Geometry: final body of the model. Coordinates: model frame, mm. A direction names the side the tool comes from. Coordinates: 2 decimals unless noted, no trailing zeros. Order: outer loops, then holes, each group sorted by start corner. A loop starts at its lowest first (then second) coordinate and runs counter-clockwise, first axis right, second up. Notation, with made-up numbers: M 42,67.25 L 82,67.25 A5 ccw 82,76.25 Z; hole C 35.5,42 d7. An arc over 180 degrees is marked long. Write item = value, one per line.
Autodesk Inventor part; units mm, degrees
ref_plane "YZ Plane" through (0, 0, 0) normal (1, 0, 0) x (0, 1, 0)
ref_plane "XZ Plane" through (0, 0, 0) normal (0, 1, 0) x (-1, 0, 0)
ref_plane "XY Plane" through (0, 0, 0) normal (0, 0, 1) x (1, 0, 0)
sketch "Sketch1" plane through (0, 0, 0) normal (0, 0, 1) x (1, 0, 0)
  line L0 (0, 70) -> (80, 70)
  line L1 (80, 70) -> (80, -70)
  line L2 (80, -70) -> (0, -70)
  line L3 (0, -70) -> (0, 70)
  line L4 (40, 70) -> (40, -70) construction
  line L5 (50, 70) -> (80, 40)
  line L6 (80, -40) -> (50, -70)
  point P0 (0, 0)
  point P1 (0, 0)
  dimension "d1" = 140
  dimension "d15" = 30
  dimension "d27" = 80
  dimension "d28" = 45
extrude "Plate1" add sketch "Sketch1" along normal blind 6 contours L0 L5 L1 L6 L2 L3
sketch "Sketch3" plane through (6, -70, 0) normal (-1, 0, 0) x (0, -1, 0)
  line L0 (-140, 0) -> (0, 0)
  line L1 (0, 0) -> (0, 60)
  line L2 (0, 60) -> (-140, 60)
  line L3 (-140, 60) -> (-140, 0)
edge flange "Flange1" height 60 angle 90 thickness 6 bend radius 6 thickness toward (-1, 0, 0) relief tear relief width 6 relief depth 3 edges at (0, 0, 6) wall of the first edge with corners at (6, 70, 0) (6, -70, 0) (6, -70, 60) (6, 70, 60)
bend "Bend1"
corner "Corner1"
equation "\"d2\" = Thickness"
equation "\"d17\" = BendReliefWidth"
equation "\"d18\" = BendReliefDepth"
equation "\"d19\" = MinimumRemnant"
equation "\"d20\" = TransitionRadius"
equation "\"d23\" = BendRadius"
equation "\"d24\" = CornerReliefSize"
equation "\"d25\" = GapSize"
equation "\"d26\" = JacobiRadiusSize"
equation "\"BendRadius\" = Thickness"
equation "\"BendReliefWidth\" = Thickness"
equation "\"BendReliefDepth\" = 0.5 * Thickness"
equation "\"CornerReliefSize\" = 4 * Thickness"
equation "\"MinimumRemnant\" = 2 * Thickness"
equation "\"TransitionRadius\" = BendRadius"
equation "\"JacobiRadiusSize\" = BendRadius"
equation "\"GapSize\" = Thickness"
properties part number "PNS-0812 floor ring  strengthen"
1) Section C-C, the plane z = 46. Return loops of the section in (x, y).
Numbers:
outline = M 0,-70 L 6,-70 L 6,70 L 0,70 Z
2) Set-up query: faces 1 (the face through (65, 55, 3)), 2 (the face through (6, -1, 36)). Return all of +Z, -Z, +X, -X, +Y, -Y with unobstructed straight access to the full face (end or side cutting, diameter ignored); none if empty.
Numbers:
face_1 = +Z, -Z, +X, +Y
face_2 = +Z, +X, +Y, -Y
3) Section B-B, the plane x = 46. Return loops of the section in (y, z), and give its area (3 significant figures).
Numbers:
outline = M -70,0 L 70,0 L 70,6 L -70,6 Z
area = 840 mm²
4) Pin query (flat end, axial travel): pin 1 (4 mm diameter, centred on y = -15, z = 50.5, fed in from +X); pin 2 (5 mm diameter, centred on x = 19.5, y = -28, fed in from +Z). Return the tip coordinate at first contact, or that it passes through.
Numbers:
pin_1 = 6
pin_2 = 6
5) Section A-A, the plane y = -24.5. Return loops of the section in (x, z).
Numbers:
outline = M 0,12 A12 ccw 12,0 L 80,0 L 80,6 L 12,6 A6 cw 6,12 L 6,60 L 0,60 Z
6) Section D-D, the plane y = 54.5. Return loops of the section in (x, z).
Numbers:
outline = M 0,12 A12 ccw 12,0 L 65.5,0 L 65.5,6 L 12,6 A6 cw 6,12 L 6,60 L 0,60 Z
7) Line query: L1, parallel to Z at x = 68.5, y = -3; L2, parallel to X at y = -29, z = 5.5. Output: solid intervals per line, ascending.
Numbers:
L1 = 0 to 6
L2 = 1.91 to 80
